```python
from build123d import *

# Parameters (mm, degrees)
SKETCH2_W           = 80
SKETCH2_H           = 80
BOSS_EXTRUDE1_DEPTH = 5
SKETCH3_R           = 8
BOSS_EXTRUDE2_DEPTH = 10.5
CUT_EXTRUDE3_DEPTH  = 3.5
SKETCH8_R           = 3.5
CUT_EXTRUDE5_DEPTH  = 67.379590237
SKETCH9_R           = 2.5
BOSS_EXTRUDE3_DEPTH = 5
SKETCH10_R          = 1.41
CUT_EXTRUDE6_DEPTH  = 61.340699366


with BuildPart() as part:
    # Sketch2 → Boss-Extrude1 (new body)
    with BuildSketch(Plane(origin=(0, 0, 0), x_dir=(1, 0, 0), z_dir=(0, 1, 0))):
        Rectangle(SKETCH2_W, SKETCH2_H)
    extrude(amount=BOSS_EXTRUDE1_DEPTH)

    # Sketch3 → Boss-Extrude2 (add, symmetric)
    with BuildSketch(Plane(origin=(0, 0, 0), x_dir=(0, 0, -1), z_dir=(1, 0, 0))):
        with Locations((0, 8)):
            Circle(SKETCH3_R)
    extrude(amount=BOSS_EXTRUDE2_DEPTH, both=True)

    # Sketch4 → Cut-Extrude3 (cut, symmetric)
    with BuildSketch(Plane(origin=(0, 0, 0), x_dir=(0, 0, -1), z_dir=(1, 0, 0))):
        Polygon((-114.767025478, 5), (-7.416198487, 5), (7.416198487, 5), (114.767025478, 5), (114.767025478, 219.701653982), (-114.767025478, 219.701653982), align=None)
    extrude(amount=CUT_EXTRUDE3_DEPTH, both=True, mode=Mode.SUBTRACT)

    # Sketch8 → Cut-Extrude5 (cut, through all)
    with BuildSketch(Plane(origin=(10.5, 0, 0), x_dir=(0, 0, -1), z_dir=(1, 0, 0))):
        with Locations((0, 9)):
            Circle(SKETCH8_R)
    extrude(amount=-CUT_EXTRUDE5_DEPTH, mode=Mode.SUBTRACT)

    # Sketch9 → Boss-Extrude3 (add)
    with BuildSketch(Plane.XZ):
        with Locations(Location((-32.705, 32.705, 0), (0, 0, 270))):
            Circle(SKETCH9_R)
        with Locations(Location((32.705, 32.705, 0), (0, 0, 270))):
            Circle(SKETCH9_R)
        with Locations(Location((-32.705, -32.705, 0), (0, 0, 270))):
            Circle(SKETCH9_R)
        with Locations(Location((32.705, -32.705, 0), (0, 0, 270))):
            Circle(SKETCH9_R)
    extrude(amount=BOSS_EXTRUDE3_DEPTH)

    # Sketch10 → Cut-Extrude6 (cut, through all)
    with BuildSketch(Plane.XZ.offset(5)):
        with Locations(Location((-32.705, -32.705, 0), (0, 0, 270))):
            Circle(SKETCH10_R)
        with Locations(Location((-32.705, 32.705, 0), (0, 0, 270))):
            Circle(SKETCH10_R)
        with Locations(Location((32.705, 32.705, 0), (0, 0, 270))):
            Circle(SKETCH10_R)
        with Locations(Location((32.705, -32.705, 0), (0, 0, 270))):
            Circle(SKETCH10_R)
    extrude(amount=-CUT_EXTRUDE6_DEPTH, mode=Mode.SUBTRACT)


solid = part.part
```
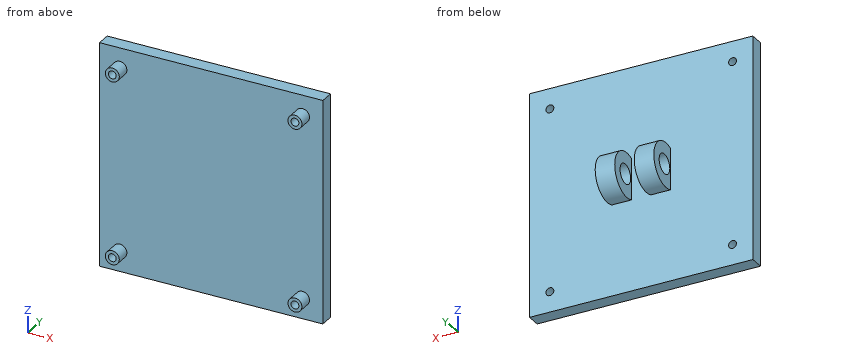
CAD build for the part. Positions are in the model's coordinates, mm. Round coordinates to 2 decimals unless told otherwise and drop trailing zeros. Order: outer loops, then holes, each group sorted by start corner. A loop starts at its lowest first (then second) coordinate and runs counter-clockwise, first axis right, second up. Notation, with made-up numbers: (23, -5.5) -> (73, -5.5) arc R15 ccw to (73, 13.5) -> close; hole circle Ø2 at (63, -10). An arc over 180 degrees is marked (long way). Write item = value, one per line.
(1) Cut at A-A (z = 0). Write the cut outline in (x, y).
Answers follow:
outline = (-40, 0) -> (40, 0) -> (40, 5) -> (10.5, 5) -> (10.5, 5.5) -> (3.5, 5.5) -> (3.5, 5) -> (-3.5, 5) -> (-3.5, 5.5) -> (-10.5, 5.5) -> (-10.5, 5) -> (-40, 5) -> close; (-10.5, 12.5) -> (-3.5, 12.5) -> (-3.5, 16) -> (-10.5, 16) -> close; (3.5, 12.5) -> (10.5, 12.5) -> (10.5, 16) -> (3.5, 16) -> close
(2) Drill centre lines: L1, parallel to Y at x = -13, z = -1.5; L2, parallel to Z at x = -6, y = 12; L3, parallel to Y at x = 5, z = -2. Where is each one in solid material? Low to high.
Answers follow:
L1 = 0 to 5
L2 = -6.93 to -1.8, 1.8 to 6.93
L3 = 0 to 6.13, 11.87 to 15.75
(3) Cut at C-C (y = 9). Write the cut outline in (x, z), plus the area to 3 significant figures.
Answers follow:
outline = (-10.5, -7.94) -> (-3.5, -7.94) -> (-3.5, -3.5) -> (-10.5, -3.5) -> close; (-10.5, 3.5) -> (-3.5, 3.5) -> (-3.5, 7.94) -> (-10.5, 7.94) -> close; (3.5, -7.94) -> (10.5, -7.94) -> (10.5, -3.5) -> (3.5, -3.5) -> close; (3.5, 3.5) -> (10.5, 3.5) -> (10.5, 7.94) -> (3.5, 7.94) -> close
area = 124 mm²
(4) Cut at D-D (x = 13.5). Write the cut outline in (y, z).
Answers follow:
outline = (0, -40) -> (5, -40) -> (5, 40) -> (0, 40) -> close
(5) Cut at B-B (y = 14.25). Write the cut outline in (x, z).
Answers follow:
outline = (-10.5, -4.99) -> (-3.5, -4.99) -> (-3.5, 4.99) -> (-10.5, 4.99) -> close; (3.5, -4.99) -> (10.5, -4.99) -> (10.5, 4.99) -> (3.5, 4.99) -> close
(6) Flat gauge pins, fed straight in: P1, Ø2, axis at x = 25, z = -14.5, coming from the +Y side; P2, Ø10, axis at x = 23.5, z = 18.5, coming from the -Y side; P3, Ø3, axis at x = 32.705, z = 32.705, coming from the -Y side; P4, Ø6.5, axis at y = 9, z = 0, coming from the +X side. Where does each tip first touch, or does it go through?
Answers follow:
P1 = 5
P2 = 0
P3 = -5
P4 = through
